Can you work these out from the drawing? Everything is in mm from the part's minimum corner. A direction names the side the tool comes from. Round coordinates to 2 decimals unless told otherwise and drop trailing zeros. Order: outer loops, then holes, each group sorted by start corner. A loop starts at its lowest first (then second) coordinate and runs counter-clockwise, first axis right, second up. Notation, with made-up numbers: M 2,77.5 L 36,77.5 A8 ccw 36,82.5 Z; hole C -30.5,86 d10. An arc over 180 degrees is marked long. Write each question's results on one line, items separated by ' | '. Start each with the question number.
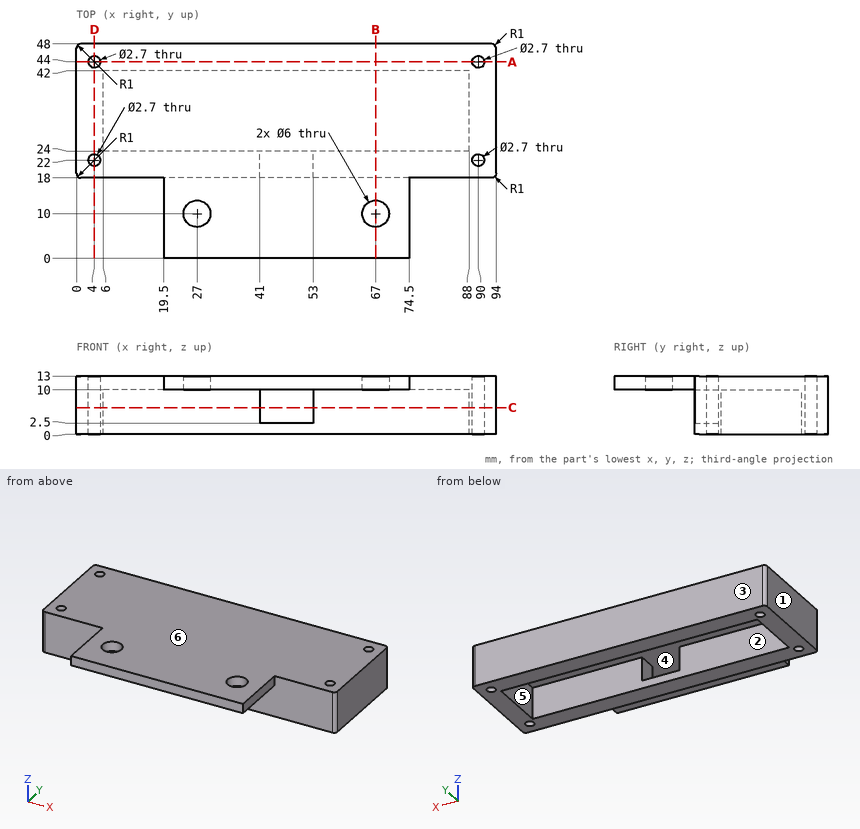
(1) I want a section at C-C on z = 6. Write out the boundary of the cut face in (x, y), and give its area (3 significant figures).
(2) Please list where these lines run through material, in increasing order: line 1 (Y direction, x = 4, z = 7.25); line 2 (Y direction, x = 12, z = 0.5); line 3 (X direction, y = 19.5, z = 7.5).
(3) I want a section at A-A on y = 44. Write out the boundary of the cut face in (x, z), and give its area (3 significant figures).
(4) I want a section at B-B on x = 67. Write out the boundary of the cut face in (y, z), and give its area (3 significant figures).
(5) I want a section at D-D on x = 4. Write out the boundary of the cut face in (y, z).
(6) On a 3-axis mill with a long thin cutter (end or side, diameter ignored), from which of +Z, -Z, +X, -X, +Y, -Y can I reach the whole of each face in a straight line? I mean the marked faces 5 and 6. Say none if no direction works.
(7) I'm going to push flat-ended pins straight in: pin 1 Ø6.5 at (x, z) = (34.5, 3.5) entering from -Y; pin 2 Ø1.5 at (y, z) = (10, 11.5) entering from +X; pin 3 Ø1.5 at (x, y) = (10.5, 30.5) entering from -Z. Where does each tip first touch, or does it pass through?
(8) If we mould it in two halves opening along X, with no side actions, what happens to the marked faces 1, 2, 3 and 4? For each: pulls with the +X half, pulls with the -X half, needs draft (parallel to the pull), parting line crosses it, or undercut.
Solutions:
1) outline: M 0,19 A1 ccw 1,18 L 41,18 L 41,24 L 6,24 L 6,42 L 88,42 L 88,24 L 53,24 L 53,18 L 93,18 A1 ccw 94,19 L 94,47 A1 ccw 93,48 L 1,48 A1 ccw 0,47 Z; hole C 4,22 d2.7; hole C 4,44 d2.7; hole C 90,22 d2.7; hole C 90,44 d2.7 | area: 1,250 mm^2
2) line 1: 18 to 20.65, 23.35 to 42.65, 45.35 to 48 | line 2: 18 to 24, 42 to 48 | line 3: 0 to 41, 53 to 94
3) outline: M 0,0 L 2.65,0 L 2.65,13 L 0,13 Z; M 5.35,0 L 88.65,0 L 88.65,13 L 5.35,13 Z; M 91.35,0 L 94,0 L 94,13 L 91.35,13 Z | area: 1,150 mm^2
4) outline: M 0,10 L 7,10 L 7,13 L 0,13 Z; M 13,10 L 18,10 L 18,0 L 24,0 L 24,10 L 42,10 L 42,0 L 48,0 L 48,13 L 13,13 Z | area: 246 mm^2
5) outline: M 18,0 L 20.65,0 L 20.65,13 L 18,13 Z; M 23.35,0 L 42.65,0 L 42.65,13 L 23.35,13 Z; M 45.35,0 L 48,0 L 48,13 L 45.35,13 Z
6) face 5: -Z | face 6: +Z, +X, -X, +Y, -Y
7) pin 1: y = 18 | pin 2: x = 74.5 | pin 3: z = 10
8) face 1: pulls with the -X half | face 2: undercut | face 3: needs draft | face 4: undercut
